The listing builds one solid part. Answer for the finished solid, in the listing's coordinates (mm). Face numbers are marked on the shaded views. Coordinates: 2 decimals unless noted, no trailing zeros. Order: outer loops, then holes, each group sorted by start corner. A loop starts at its lowest first (then second) coordinate and runs counter-clockwise, first axis right, second up. Notation, with made-up numbers: M 11,55 L 54,55 A26 cw 54,75 Z; hole C -11.5,-8.75 d8. An arc over 180 degrees is marked long. One line per item, written item: value. Start each with the question number.
Q1. Determine the mould class of the marked faces 1 and 2 for opening direction Z: pulls with the +Z half, pulls with the -Z half, needs draft (parallel to the pull), parting line crosses it, or undercut.
Q2. Each of these flat-tipped pins is pushed along its axis until it touches: pin 1 Ø20 at (x, y) = (4, 46.5) entering from +Z; pin 2 Ø2 at (x, y) = (-11.5, 22) entering from -Z; pin 3 Ø5 at (x, z) = (-58, 35) entering from +Y. Where does it stop, or does it pass through?
Q3. The part is cut by section B-B on x = 58. Give the vertices of the cut face in (y, z).
Q4. The part is cut by section A-A on z = -75. Give the vertices of the cut face in (x, y), then the cut area to 3 significant figures.
Q5. The part is cut by section C-C on y = 71. Give the vertices of the cut face in (x, z).
Q6. Straight lines are drawn through the part: line 1 along X through (y, z) = (3, 35); line 2 along X through (y, z) = (4, -25); line 3 along Z through (x, y) = (58, 4). For each, find the intervals that lie inside material, in ascending order. Write a range as [from, to].
Q7. The part is cut by section D-D on z = 9.5. Give the vertices of the cut face in (x, y), then the cut area to 3 significant figures.
```python
from build123d import *

# Parameters (mm, degrees)
BOSS_EXTRUDE1_DEPTH = 7
BOSS_EXTRUDE2_DEPTH = 80
CUT_EXTRUDE1_DEPTH  = 28
SKETCH4_W           = 8
SKETCH4_H           = 1.100013063
CUT_EXTRUDE2_DEPTH  = 88
SKETCH5_W           = 25
SKETCH5_H           = 80
BOSS_EXTRUDE3_DEPTH = 6.2
SKETCH8_R           = 2.1
CUT_EXTRUDE3_DEPTH  = 6
SKETCH13_W          = 25
SKETCH13_H          = 74
CUT_EXTRUDE11_DEPTH = 6
SKETCH15_W          = 8.5
SKETCH15_H          = 6
BOSS_EXTRUDE6_DEPTH = 6.2
SKETCH16_R          = 2.1
CUT_EXTRUDE12_DEPTH = 6.2
SKETCH17_R          = 2.15
CUT_EXTRUDE13_DEPTH = 8
SKETCH18_W          = 76
SKETCH18_H          = 10
CUT_EXTRUDE14_DEPTH = 8


with BuildPart() as part:
    # Sketch1 → Boss-Extrude1 (new body)
    with BuildSketch(Plane(origin=(0, 0, 0), x_dir=(1, 0, 0), z_dir=(0, 1, 0))):
        Polygon((-72.5, -85), (72.5, -85), (72.5, 85), (12.5, 85), (-12.5, 85), (-72.5, 85), align=None)
    extrude(amount=BOSS_EXTRUDE1_DEPTH)

    # Sketch2 → Boss-Extrude2 (add)
    with BuildSketch(Plane(origin=(0, 7, 0), x_dir=(1, 0, 0), z_dir=(0, 1, 0))):
        Polygon((12.5, 21.999959178), (-12.5, 22), (-12.499999895, -22), (12.500000105, -22.000040822), align=None)
    extrude(amount=BOSS_EXTRUDE2_DEPTH)

    # Sketch3 → Cut-Extrude1 (cut)
    with BuildSketch(Plane(origin=(0, 87, 0), x_dir=(1, 0, 0), z_dir=(0, 1, 0))):
        Polygon((-11.399999997, 20.899998204), (-11.399999897, -20.900001796), (11.400000102, -20.900039025), (11.400000003, 20.899960975), align=None)
    extrude(amount=-CUT_EXTRUDE1_DEPTH, mode=Mode.SUBTRACT)

    # Sketch4 → Cut-Extrude2 (cut, through all)
    with BuildSketch(Plane(origin=(0, 87, 0), x_dir=(1, 0, 0), z_dir=(0, 1, 0))):
        with Locations((0, 21.44997959)):
            Rectangle(SKETCH4_W, SKETCH4_H)
    extrude(amount=-CUT_EXTRUDE2_DEPTH, mode=Mode.SUBTRACT)

    # Sketch5 → Boss-Extrude3 (add)
    with BuildSketch(Plane(origin=(-3.5923e-05, 0, 22.000020411), x_dir=(1, 0, 1.633e-06), z_dir=(-1.633e-06, 0, 1))):
        with Locations((3.6028e-05, 47)):
            Rectangle(SKETCH5_W, SKETCH5_H)
    extrude(amount=BOSS_EXTRUDE3_DEPTH)

    # Sketch8 → Cut-Extrude3 (cut)
    with BuildSketch(Plane(origin=(0, 87, 0), x_dir=(1, 0, 0), z_dir=(0, 1, 0))):
        with Locations((5.700000051, -24.900029718)):
            Circle(SKETCH8_R)
        with Locations((-5.700000051, -24.900029718)):
            Circle(SKETCH8_R)
    extrude(amount=-CUT_EXTRUDE3_DEPTH, mode=Mode.SUBTRACT)

    # Sketch13 → Cut-Extrude11 (cut)
    with BuildSketch(Plane(origin=(-4.6047e-05, 0, 28.200020411), x_dir=(1, 0, 1.633e-06), z_dir=(-1.633e-06, 0, 1))):
        with Locations((3.6028e-05, 44)):
            Rectangle(SKETCH13_W, SKETCH13_H)
    extrude(amount=-CUT_EXTRUDE11_DEPTH, mode=Mode.SUBTRACT)

    # Sketch15 → Boss-Extrude6 (add)
    with BuildSketch(Plane(origin=(3.5923e-05, 0, -21.999979589), x_dir=(-1, 0, -1.633e-06), z_dir=(1.633e-06, 0, -1))):
        with Locations((-8.249964077, 84)):
            Rectangle(SKETCH15_W, SKETCH15_H)
        with Locations((8.249964077, 84)):
            Rectangle(SKETCH15_W, SKETCH15_H)
    extrude(amount=BOSS_EXTRUDE6_DEPTH)

    # Sketch16 → Cut-Extrude12 (cut)
    with BuildSketch(Plane(origin=(0, 87, 0), x_dir=(1, 0, 0), z_dir=(0, 1, 0))):
        with Locations((5.700000051, -24.900029718)):
            Circle(SKETCH16_R)
        with Locations((-5.700000051, -24.900029718)):
            Circle(SKETCH16_R)
        with Locations((5.700000051, 24.900029718)):
            Circle(SKETCH16_R)
        with Locations((-5.700000051, 24.900029718)):
            Circle(SKETCH16_R)
    extrude(amount=-CUT_EXTRUDE12_DEPTH, mode=Mode.SUBTRACT)

    # Sketch17 → Cut-Extrude13 (cut, through all)
    with BuildSketch(Plane(origin=(0, 7, 0), x_dir=(1, 0, 0), z_dir=(0, 1, 0))):
        with Locations((-58, 75)):
            Circle(SKETCH17_R)
        with Locations((-58, 25)):
            Circle(SKETCH17_R)
        with Locations((-58, -35)):
            Circle(SKETCH17_R)
        with Locations((58, -35)):
            Circle(SKETCH17_R)
        with Locations((58, 25)):
            Circle(SKETCH17_R)
        with Locations((58, 75)):
            Circle(SKETCH17_R)
    extrude(amount=-CUT_EXTRUDE13_DEPTH, mode=Mode.SUBTRACT)

    # Sketch18 → Cut-Extrude14 (cut, through all)
    with BuildSketch(Plane(origin=(0, 7, 0), x_dir=(1, 0, 0), z_dir=(0, 1, 0))):
        with Locations((0, 30.200020411)):
            Rectangle(SKETCH18_W, SKETCH18_H)
        with Locations((0, -30.200020411)):
            Rectangle(SKETCH18_W, SKETCH18_H)
    extrude(amount=-CUT_EXTRUDE14_DEPTH, mode=Mode.SUBTRACT)


solid = part.part
```
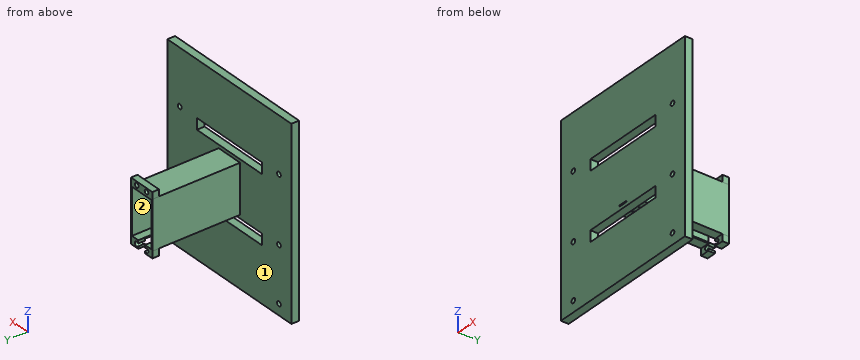
Output:
1. face 1: needs draft
1. face 2: undercut
2. pin 1: stops at z = 22.2
2. pin 2: stops at z = -22
2. pin 3: stops at y = 7
3. outline: M 0,-85 L 7,-85 L 7,-77.15 L 0,-77.15 Z; M 0,-72.85 L 7,-72.85 L 7,-27.15 L 0,-27.15 Z; M 0,-22.85 L 7,-22.85 L 7,32.85 L 0,32.85 Z; M 0,37.15 L 7,37.15 L 7,85 L 0,85 Z
4. outline: M -72.5,0 L -60.15,0 L -60.15,7 L -72.5,7 Z; M -55.85,0 L 55.85,0 L 55.85,7 L -55.85,7 Z; M 60.15,0 L 72.5,0 L 72.5,7 L 60.15,7 Z
4. area: 955 mm^2
5. outline: M -12.5,-22 L -4,-22 L -4,-20.9 L -11.4,-20.9 L -11.4,20.9 L 11.4,20.9 L 11.4,-20.9 L 4,-20.9 L 4,-22 L 12.5,-22 L 12.5,22 L 12.5,22.2 L -12.5,22.2 L -12.5,22 Z
6. line 1: x = [-72.5, -60.15], [-55.85, -38], [38, 55.85], [60.15, 72.5]
6. line 2: x = [-72.5, -60.15], [-55.85, 55.85], [60.15, 72.5]
6. line 3: z = [-85, -77.15], [-72.85, -27.15], [-22.85, 32.85], [37.15, 85]
7. outline: M -72.5,0 L 72.5,0 L 72.5,7 L 12.5,7 L 12.5,87 L 11.4,87 L 11.4,59 L -11.4,59 L -11.4,87 L -12.5,87 L -12.5,7 L -72.5,7 Z
7. area: 2,380 mm^2
